from build123d import *

# Parameters (mm, degrees)
BOSS_EXTRUDE1_DEPTH = 7
FILLET1_R           = 3
SKETCH3_W           = 34.7
SKETCH3_H           = 20
SKETCH3_R           = 1.5
BOSS_EXTRUDE2_DEPTH = 4


with BuildPart() as part:
    # Sketch1 → Boss-Extrude1 (new body)
    with BuildSketch(Plane.XY):
        Polygon((7, 0), (34.7, 0), (34.7, 9), (0, 9), (0, 0), (0, -26.65), (-6, -26.65), (-6, -29.15), (0, -29.15), (7, -29.15), align=None)
    extrude(amount=BOSS_EXTRUDE1_DEPTH)

    # Fillet1
    fillet1_edges = [part.edges().sort_by_distance(p)[0] for p in [
        (7, 0, 3.5),
        (7, -29.15, 3.5),
        (0, -26.65, 3.5),
    ]]
    fillet(fillet1_edges, radius=FILLET1_R)

    # Sketch3 → Boss-Extrude2 (add)
    with BuildSketch(Plane(origin=(0, 9, 0), x_dir=(1, 0, 0), z_dir=(0, 1, 0))):
        with Locations((17.35, -10)):
            Rectangle(SKETCH3_W, SKETCH3_H)
        with Locations(Location((24.85, -15, 0), (0, 0, 270))):
            Circle(SKETCH3_R, mode=Mode.SUBTRACT)
        with Locations(Location((9.85, -15, 0), (0, 0, 270))):
            Circle(SKETCH3_R, mode=Mode.SUBTRACT)
    extrude(amount=BOSS_EXTRUDE2_DEPTH)


solid = part.part
For this review, take the finished solid that the model builds, in its own axes (mm). A direction names the side the tool comes from. Round coordinates to 2 decimals unless told otherwise and drop trailing zeros. Loops run counter-clockwise (first coordinate to the right, second up) from the corner with the lowest first, then second, coordinate; pieces in that order, holes last. Notation, with made-up numbers: (-39, 9.5) - (-24, 9.5) arc R25 ccw to (-24, 37.5) - close; hole circle Ø3 at (45, 1.5). An arc over 180 degrees is marked (long way). One line per question, with ' | ' between items.
Q1. Take a section at B-B (x = 24.85). Give the boundary of the cut face in (y, z), and give its area (3 significant figures).
Taken from the geometry:
outline: (0, 0) - (13, 0) - (13, 13.5) - (9, 13.5) - (9, 7) - (0, 7) - close; (9, 16.5) - (13, 16.5) - (13, 20) - (9, 20) - close | area: 131 mm²
Q2. Take a section at A-A (z = 15). Give the boundary of the cut face in (x, y), and give its area (3 significant figures).
Taken from the geometry:
outline: (0, 9) - (8.35, 9) - (8.35, 13) - (0, 13) - close; (11.35, 9) - (23.35, 9) - (23.35, 13) - (11.35, 13) - close; (26.35, 9) - (34.7, 9) - (34.7, 13) - (26.35, 13) - close | area: 115 mm²
Q3. For pin 1 (8 mm diameter, centred on x = 26.5, z = 18, fed in from -Y); pin 2 (2.5 mm diameter, centred on x = 24.85, z = 15, fed in from -Y); pin 3 (3.5 mm diameter, centred on x = -4.5, z = 3.5, fed in from +Y); pin 4 (7.5 mm diameter, centred on y = -10.5, z = 2.5, fed in from +X), all flat-tipped, find the tip position at first contact; note any pin that passes through.
Taken from the geometry:
pin 1: stops at y = 9 | pin 2: passes through | pin 3: stops at y = -26.64 | pin 4: stops at x = 7
Q4. Take a section at C-C (z = 1.5). Give the boundary of the cut face in (x, y).
Taken from the geometry:
outline: (-6, -29.15) - (4, -29.15) arc R3 ccw to (7, -26.15) - (7, -3) arc R3 cw to (10, 0) - (34.7, 0) - (34.7, 13) - (0, 13) - (0, -23.65) arc R3 cw to (-3, -26.65) - (-6, -26.65) - close
Q5. Tool access review of faces 1 (the flat face through (5, -6, 7)), 2 (the flat face through (22, 0, 3)), 3 (the flat face through (-4, -26.65, 3)), 4 (the flat face through (-1, -29.15, 3)): name each direction out of +Z, -Z, +X, -X, +Y, -Y from which nothing blocks a thin tool from reaching the whole face with its end or side.
Taken from the geometry:
face 1: +Z, +X, -X, -Y | face 2: +Z, -Z, +X, -Y | face 3: +Z, -Z, -X, +Y | face 4: +Z, -Z, +X, -X, -Y
Q6. The part is to be moulded in two halves that separate along X. For faces 5 (the cylindrical face through (10.86, 10.97, 13.89)), 6 (the flat face through (7, -15, 3)), 7 (the cylindrical face through (25.86, 10.97, 13.89)), 8 (the flat face through (17, 9, 13)), say which applies: released by +X, released by -X, zero draft, split by the parting line, or undercut.
Taken from the geometry:
face 5: undercut | face 6: released by +X | face 7: undercut | face 8: zero draft
Q7. For line 1 along X through (y, z) = (9.9, 15); line 2 along Z through (x, y) = (4, -15); line 3 along Y through (x, z) = (12, 18.75), list the stretches that pass through material, from the lowest coordinate up. Write a range as [from, to].
Taken from the geometry:
line 1: x = [0, 8.35], [11.35, 23.35], [26.35, 34.7] | line 2: z = [0, 7] | line 3: y = [9, 13]
Q8. Take a section at D-D (y = -5). Give the boundary of the cut face in (x, z), and give its area (3 significant figures).
Taken from the geometry:
outline: (0, 0) - (7, 0) - (7, 7) - (0, 7) - close | area: 49.0 mm²
